from build123d import *

# Parameters (mm, degrees)
F1_DEPTH = 3


with BuildPart() as f1:
    # F0 (on Front) → F1 (new body)
    with BuildSketch(Plane.XZ):
        with BuildLine():
            ThreePointArc((0, 40), (-6.189391, 37.85439), (-9.722778, 32.338287))
            Line((-9.722778, 32.338287), (-17.5, 0))
            Line((-17.5, 0), (-7.5, 0))
            Line((-7.5, 0), (-7.5, -3))
            Line((-7.5, -3), (0, -3))
            Line((0, -3), (7.5, -3))
            Line((7.5, -3), (7.5, 0))
            Line((7.5, 0), (17.5, 0))
            Line((17.5, 0), (9.722778, 32.338287))
            ThreePointArc((9.722778, 32.338287), (6.189391, 37.85439), (0, 40))
        make_face()
        with BuildLine():
            ThreePointArc((0, 23.5), (-6.5, 30), (0, 36.5))
            ThreePointArc((0, 36.5), (6.5, 30), (0, 23.5))
        make_face(mode=Mode.SUBTRACT)
    extrude(amount=F1_DEPTH)


solid = f1.part
Source: CAD feature listing. Evaluate the final solid. Frame: model axes, mm. A direction names the side the tool comes from. Round coordinates to 2 decimals unless told otherwise and drop trailing zeros. Loops run counter-clockwise (first coordinate to the right, second up) from the corner with the lowest first, then second, coordinate; pieces in that order, holes last. Notation, with made-up numbers: M 0,71.25 L 35,71.25 A8 cw 35,79.25 Z; hole C 58,-29.75 d10. An arc over 180 degrees is marked long. Return JSON: item names as keys, results as strings. Group by question number.
1. Mould query, pull axis X, two halves, no side actions, for faces 1 (the face through (12, -1, 0)), 2 (the face through (0.286, -1.479, 23.506)), 3 (the face through (-13.557, -1.479, 16.396)), 4 (the face through (13.666, -1.479, 15.943)). Classes: released by +X, released by -X, zero draft, split by the parting line, or undercut.
2. Material intervals for line 1 along Z through (x, y) = (0.5, -2.15); line 2 along X through (y, z) = (-0.65, 25); line 3 along Z through (x, y) = (6, -2.8), sorted ascending. Write a range as from..to.
3. Reachability of faces 5 (the face through (-7.5, -1, -1)), 6 (the face through (7.5, -1, -2)), 7 (the face through (0, -1, -3)) from +Z, -Z, +X, -X, +Y, -Y: full face, straight path, thin tool, end or side. Return the list, or none.
4. Pin query (flat end, axial travel): pin 1 (0.9 mm diameter, centred on y = -1.5, z = -1, fed in from +X); pin 2 (0.9 mm diameter, centred on x = -13, y = -2, fed in from -Z); pin 3 (11.5 mm diameter, centred on x = 0, z = 30, fed in from -Y). Return the tip coordinate at first contact, or that it passes through.
5. Section query D-D on z = 9. Output: boundary loops of the cut face in (x, y).
6. Section query A-A on y = -0.5. Output: boundary loops of the cut face in (x, z), and give its area (3 significant figures).
7. Section query C-C on z = 29. Output: boundary loops of the cut face in (x, y).
8. Section query B-B on x = 3.5. Output: boundary loops of the cut face in (y, z), and give its area (3 significant figures).
Checks:
{
 "1": {"face 1": "zero draft", "face 2": "undercut", "face 3": "released by -X", "face 4": "released by +X"},
 "2": {"line 1": "z = -3..23.52, 36.48..39.99", "line 2": "x = -11.49..-4.15, 4.15..11.49", "line 3": "z = -3..27.5, 32.5..38"},
 "3": {"face 5": "-Z, -X, +Y, -Y", "face 6": "-Z, +X, +Y, -Y", "face 7": "-Z, +X, -X, +Y, -Y"},
 "4": {"pin 1": "stops at x = 7.5", "pin 2": "stops at z = 0", "pin 3": "passes through"},
 "5": {"outline": "M -15.34,-3 L 15.34,-3 L 15.34,0 L -15.34,0 Z"},
 "6": {"outline": "M -17.5,0 L -7.5,0 L -7.5,-3 L 7.5,-3 L 7.5,0 L 17.5,0 L 9.72,32.34 A10 ccw 0,40 A10 ccw -9.72,32.34 Z; hole C 0,30 d13", "area": "903 mm²"},
 "7": {"outline": "M -10.53,-3 L -6.42,-3 L -6.42,0 L -10.53,0 Z; M 6.42,-3 L 10.53,-3 L 10.53,0 L 6.42,0 Z"},
 "8": {"outline": "M -3,-3 L 0,-3 L 0,24.52 L -3,24.52 Z; M -3,35.48 L 0,35.48 L 0,39.37 L -3,39.37 Z", "area": "94.2 mm²"}
}
